The model under review builds one solid part; all positions refer to its coordinate system, in mm. Face numbers are marked on the shaded views. Coordinates: 2 decimals unless noted, no trailing zeros. Order: outer loops, then holes, each group sorted by start corner. A loop starts at its lowest first (then second) coordinate and runs counter-clockwise, first axis right, second up.
```python
from build123d import *

# Parameters (mm, degrees)
BOSS_EXTRUDE1_DEPTH = 12
BOSS_EXTRUDE2_DEPTH = 3.2
BOSS_EXTRUDE3_DEPTH = 3
SKETCH6_R           = 16
BOSS_EXTRUDE4_DEPTH = 35
SKETCH7_R           = 19
BOSS_EXTRUDE5_DEPTH = 57.1


with BuildPart() as part:
    # Sketch2 → Boss-Extrude1 (new body)
    with BuildSketch(Plane(origin=(0, 0, 0), x_dir=(1, 0, 0), z_dir=(0, 1, 0))):
        with BuildLine():
            Line((2.75, 1.198957881), (-2.75, 1.198957881))
            ThreePointArc((-2.75, 1.198957881), (-0.612372436, -2.936835031), (3, 0))
            ThreePointArc((3, 0), (2.936835031, 0.612372436), (2.75, 1.198957881))
        make_face()
    extrude(amount=BOSS_EXTRUDE1_DEPTH)

    # Sketch3 → Boss-Extrude2 (add)
    with BuildSketch(Plane(origin=(0, 12, 0), x_dir=(1, 0, 0), z_dir=(0, 1, 0))):
        with BuildLine():
            Line((2.75, 1.198957881), (-2.75, 1.198957881))
            ThreePointArc((-2.75, 1.198957881), (-0.612372436, -2.936835031), (3, 0))
            ThreePointArc((3, 0), (2.936835031, 0.612372436), (2.75, 1.198957881))
        make_face()
        with BuildLine():
            ThreePointArc((2.75, 1.198957881), (0, 3), (-2.75, 1.198957881))
            Line((-2.75, 1.198957881), (2.75, 1.198957881))
        make_face()
        with BuildLine():
            ThreePointArc((-2.75, 1.198957881), (0, -3), (2.75, 1.198957881))
            Line((2.75, 1.198957881), (-2.75, 1.198957881))
        make_face()
    extrude(amount=BOSS_EXTRUDE2_DEPTH)

    # Sketch5 → Boss-Extrude3 (add)
    with BuildSketch(Plane(origin=(0, 15.2, 0), x_dir=(1, 0, 0), z_dir=(0, 1, 0))):
        with BuildLine():
            Line((-9, 4.358898944), (-9, -4.358898944))
            ThreePointArc((-9, -4.358898944), (0, -10), (9, -4.358898944))
            Line((9, -4.358898944), (9, 4.358898944))
            ThreePointArc((9, 4.358898944), (0, 10), (-9, 4.358898944))
        make_face()
    extrude(amount=BOSS_EXTRUDE3_DEPTH)

    # Sketch6 → Boss-Extrude4 (add)
    with BuildSketch(Plane(origin=(0, 18.2, 0), x_dir=(1, 0, 0), z_dir=(0, 1, 0))):
        Circle(SKETCH6_R)
    extrude(amount=BOSS_EXTRUDE4_DEPTH)

    # Sketch7 → Boss-Extrude5 (add)
    with BuildSketch(Plane(origin=(0, 53.2, 0), x_dir=(1, 0, 0), z_dir=(0, 1, 0))):
        Circle(SKETCH7_R)
    extrude(amount=BOSS_EXTRUDE5_DEPTH)


solid = part.part
```
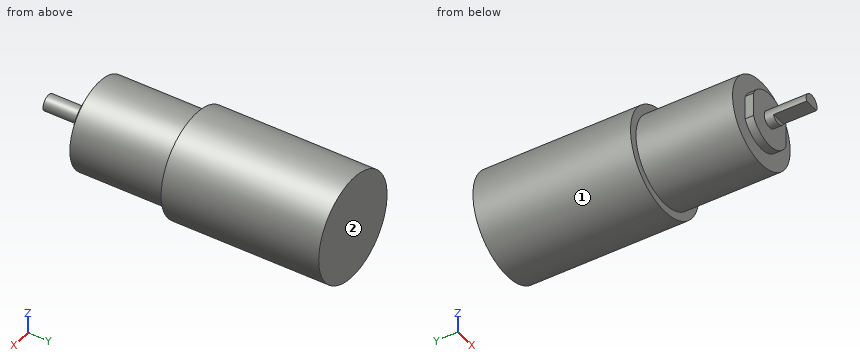
(1) We need section B-B, the plane z = 0. Write out the cut boundary in (x, y), and give its area (4 significant figures).
A:
outline: (-19, 53.2) - (-16, 53.2) - (-16, 18.2) - (-9, 18.2) - (-9, 15.2) - (-3, 15.2) - (-3, 0) - (3, 0) - (3, 15.2) - (9, 15.2) - (9, 18.2) - (16, 18.2) - (16, 53.2) - (19, 53.2) - (19, 110.3) - (-19, 110.3) - close
area: 3,435 mm2
(2) Wall thickness on probe 1 along Y at (x, z) = (-13.5, -3); probe 2 along Y at (x, z) = (6.5, -15); probe 3 along Z at (x, y) = (-0.5, 61.5): over which ranges is each line inside the solid? List them lowest first.
A:
probe 1: y = 18.2 to 110.3
probe 2: y = 53.2 to 110.3
probe 3: z = -18.99 to 18.99
(3) Draft analysis for pull direction Z (two halves, no side actions). For the marked faces 1 and 2, state which applies: released by +Z, released by -Z, zero draft, split by the parting line, or undercut.
A:
face 1: split by the parting line
face 2: zero draft
(4) We need section C-C, the plane y = 99.5. Write out the cut boundary in (x, z), and give its area (3 significant figures).
A:
outline: circle Ø38 at (0, 0)
area: 1,130 mm2
(5) For pin 1 Ø0.9 at (y, z) = (16, -2) entering from +X; pin 2 Ø1 at (x, z) = (6.5, -3) entering from -Y; pin 3 Ø12 at (x, z) = (-4, 1) entering from -Y; pin 4 Ø1.5 at (y, z) = (25, 8) entering from +X, all flat-tipped, find the tip position at first contact; note any pin that passes through.
A:
pin 1: stops at x = 9
pin 2: stops at y = 15.2
pin 3: stops at y = 0
pin 4: stops at x = 14.26
(6) We need section D-D, the plane x = 6.5. Write out the cut boundary in (y, z).
A:
outline: (15.2, -7.6) - (18.2, -7.6) - (18.2, -14.62) - (53.2, -14.62) - (53.2, -17.85) - (110.3, -17.85) - (110.3, 17.85) - (53.2, 17.85) - (53.2, 14.62) - (18.2, 14.62) - (18.2, 7.6) - (15.2, 7.6) - close
(7) We need section A-A, the plane x = 0. Write out the cut boundary in (y, z).
A:
outline: (0, -1.2) - (12, -1.2) - (12, -3) - (15.2, -3) - (15.2, -10) - (18.2, -10) - (18.2, -16) - (53.2, -16) - (53.2, -19) - (110.3, -19) - (110.3, 19) - (53.2, 19) - (53.2, 16) - (18.2, 16) - (18.2, 10) - (15.2, 10) - (15.2, 3) - (0, 3) - close
